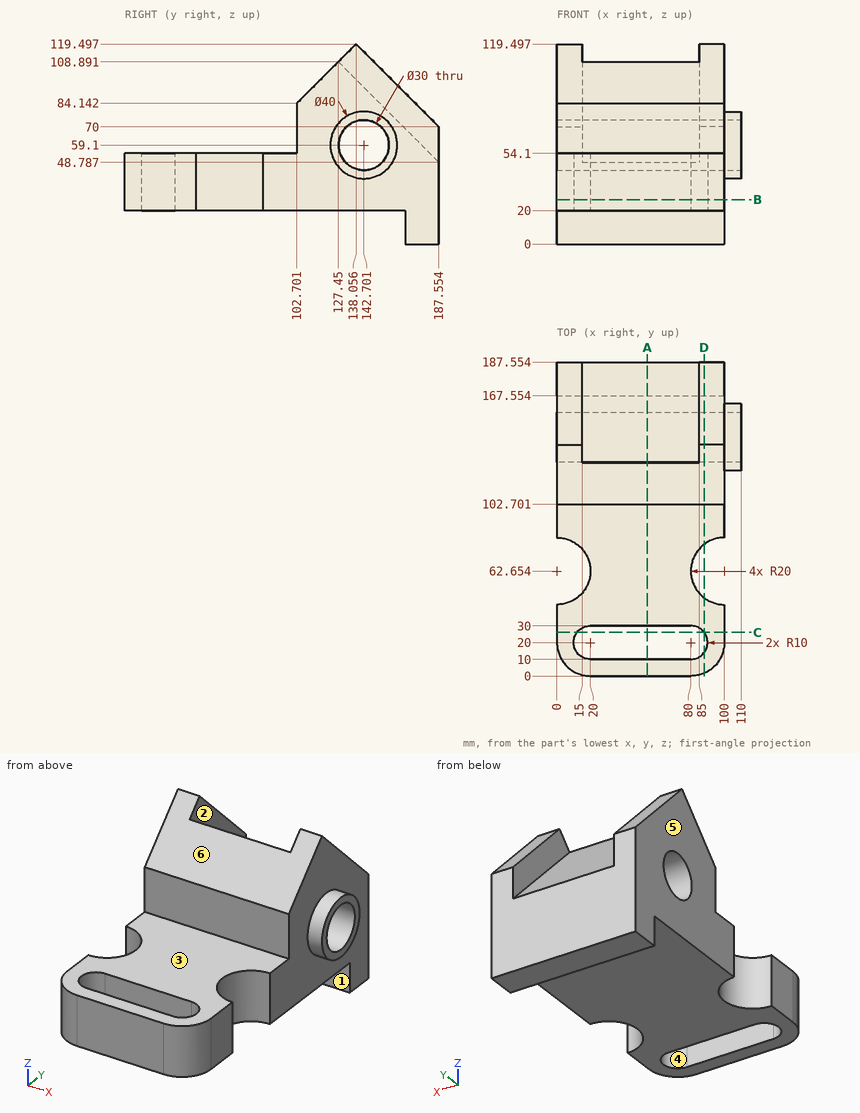
Geometry: see drawing. Coordinates: mm, zero at the bounding-box minimum. A direction names the side the tool comes from. Round coordinates to 2 decimals unless told otherwise and drop trailing zeros. Loops run counter-clockwise (first coordinate to the right, second up) from the corner with the lowest first, then second, coordinate; pieces in that order, holes last. Notation, with made-up numbers: (-40, 34.25) -> (15, 34.25) arc R6 cw to (15, 38.25) -> close; hole circle Ø11 at (79, 73.5). An arc over 180 degrees is marked (long way). Write each question's results on one line, items separated by ' | '.
1. Mould query, pull axis Y, two halves, no side actions, for the marked faces 4, 5 and 6. Classes: +Y half, -Y half, draft (parallel to the pull), parting line (faces both ways), or undercut.
Geometry results:
face 4: undercut | face 5: draft | face 6: -Y half
2. Section C-C (y = 26). Return loops of the section in (x, z).
Geometry results:
outline: (0, 20) -> (12, 20) -> (12, 54.1) -> (0, 54.1) -> close; (88, 20) -> (100, 20) -> (100, 54.1) -> (88, 54.1) -> close
3. Section B-B (z = 26.5). Return loops of the section in (x, y), and give its area (3 significant figures).
Geometry results:
outline: (0, 20) arc R20 ccw to (20, 0) -> (80, 0) arc R20 ccw to (100, 20) -> (100, 42.65) arc R20 cw to (100, 82.65) -> (100, 187.55) -> (0, 187.55) -> (0, 82.65) arc R20 cw to (0, 42.65) -> close; hole (20, 10) -> (80, 10) arc R10 ccw to (80, 30) -> (20, 30) arc R10 ccw to start | area: 15,800 mm2
4. Ray query, line 1 (Y direction, x = 51.5, z = 43); line 2 (Y direction, x = 86.5, z = 59.1); line 3 (X direction, y = 108, z = 47). Return the intervals inside material, ascending. Write a range as from..to.
Geometry results:
line 1: 0..10, 30..187.55 | line 2: 102.7..127.7, 157.7..187.55 | line 3: 0..100
5. Set-up query: the marked faces 1, 2 and 3. Return all of +Z, -Z, +X, -X, +Y, -Y with unobstructed straight access to the full face (end or side cutting, diameter ignored); none if empty.
Geometry results:
face 1: -Z, +X, -X, -Y | face 2: +Z, +Y | face 3: +Z, +X, -X, -Y
6. First-contact query: P1, Ø22, axis at x = 57, z = 7.5, coming from the -Y side; P2, Ø8, axis at y = 64.5, z = 53.5, coming from the +X side; P3, Ø24, axis at x = 40, z = 76.5, coming from the -Y side. Flat tips, straight axial feed; report the tip coordinate or a pass-through.
Geometry results:
P1: y = 167.55 | P2: x = 80.87 | P3: y = 102.7
7. Section A-A (x = 54). Return loops of the section in (y, z).
Geometry results:
outline: (0, 20) -> (10, 20) -> (10, 54.1) -> (0, 54.1) -> close; (30, 20) -> (167.55, 20) -> (167.55, 0) -> (187.55, 0) -> (187.55, 48.79) -> (127.45, 108.89) -> (102.7, 84.14) -> (102.7, 54.1) -> (30, 54.1) -> close; hole circle Ø30 at (142.7, 59.1)
8. Section D-D (x = 88). Return loops of the section in (y, z), and give its area (3 significant figures).
Geometry results:
outline: (1.67, 20) -> (14, 20) -> (14, 54.1) -> (1.67, 54.1) -> close; (26, 20) -> (46.65, 20) -> (46.65, 54.1) -> (26, 54.1) -> close; (78.65, 20) -> (167.55, 20) -> (167.55, 0) -> (187.55, 0) -> (187.55, 70) -> (138.06, 119.5) -> (102.7, 84.14) -> (102.7, 54.1) -> (78.65, 54.1) -> close; hole circle Ø30 at (142.7, 59.1) | area: 8,230 mm2
